Can you work these out from the drawing? Everything is in mm from the part's minimum corner. Coordinates: 2 decimals unless noted, no trailing zeros. Order: outer loops, then holes, each group sorted by start corner. A loop starts at its lowest first (then second) coordinate and runs counter-clockwise, first axis right, second up. Notation, with made-up numbers: (14, -24) - (19, -24) arc R15 cw to (19, -6) - close; hole circle Ø1 at (21, 89.25). An arc over 180 degrees is marked (long way). Answer as CSV lines item,"result". Start each with the question number.
Q1. Suppose I cut it at B-B (y = 70.5). Please give me the cut outline in (x, z).
Q2. Thinking about a two-plate mould opening in Z: for the marked faces 1 and 2, which applies, released by +Z, released by -Z, zero draft, split by the parting line, or undercut?
Q3. I need wall thicknesses on line 1 (Y direction, x = 149.86, z = 4.5); line 2 (X direction, y = 42.5, z = 0.75); line 3 (X direction, y = 37.5, z = 2). Which ranges of each line are inside material? Lowest first, please.
Q4. Suppose I cut it at C-C (y = 15.5). Please give me the cut outline in (x, z).
Q5. Suppose I cut it at A-A (x = 22.5). Please give me the cut outline in (y, z).
Q6. For pin 1 Ø1.3 at (y, z) = (18, 5) entering from +X; pin 2 Ø1 at (y, z) = (26, 2.5) entering from -X; pin 3 Ø0.8 at (y, z) = (59, 2) entering from +X, each with a flat end and sliding along its axis, tell me the tip position at first contact or that it passes through.
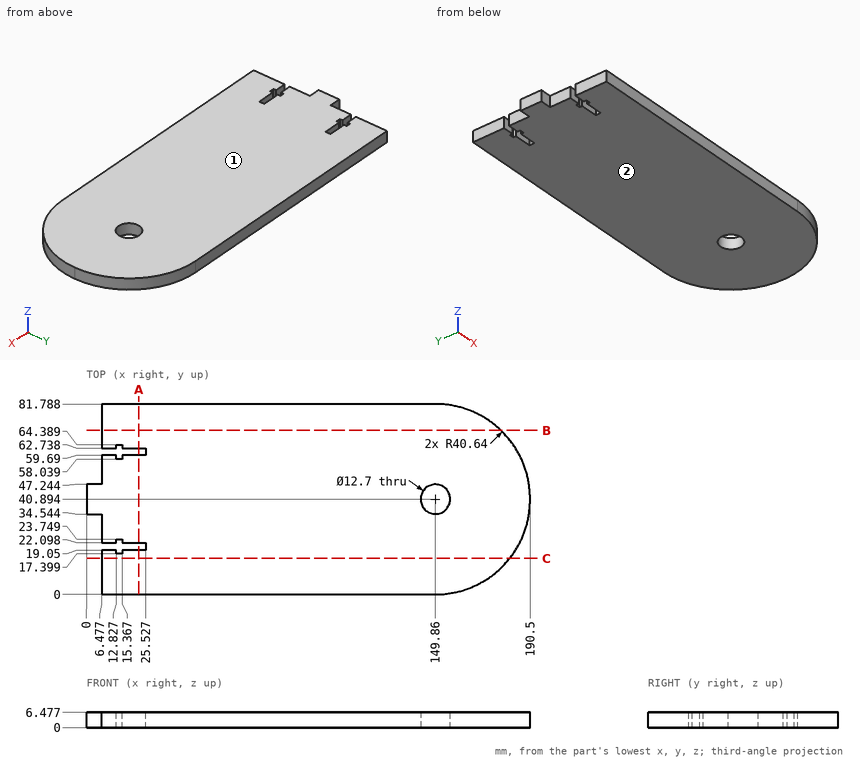
Here are the results:
1,outline,"(6.48, 0) - (177.97, 0) - (177.97, 6.48) - (6.48, 6.48) - close"
2,face 1,"released by +Z"
2,face 2,"released by -Z"
3,line 1,"y = 0 to 34.54, 47.24 to 81.79"
3,line 2,"x = 0 to 143.72, 156 to 190.48"
3,line 3,"x = 0 to 144.49, 155.23 to 190.38"
4,outline,"(6.48, 0) - (181.79, 0) - (181.79, 6.48) - (6.48, 6.48) - close"
5,outline,"(0, 0) - (19.05, 0) - (19.05, 6.48) - (0, 6.48) - close; (22.1, 0) - (59.69, 0) - (59.69, 6.48) - (22.1, 6.48) - close; (62.74, 0) - (81.79, 0) - (81.79, 6.48) - (62.74, 6.48) - close"
6,pin 1,"stops at x = 184.04"
6,pin 2,"stops at x = 6.48"
6,pin 3,"stops at x = 186.56"
